The model under review builds one solid part; all positions refer to its coordinate system, in mm. A direction names the side the tool comes from. Coordinates: 2 decimals unless noted, no trailing zeros. Order: outer loops, then holes, each group sorted by start corner. A loop starts at its lowest first (then second) coordinate and runs counter-clockwise, first axis right, second up. Notation, with made-up numbers: (63.25, -10.5) -> (94.25, -10.5) arc R19 ccw to (94.25, 25.5) -> close; hole circle Ø7 at (24.5, 88.5). An arc over 180 degrees is marked (long way). Put each result on its own line as item: value.
Autodesk Inventor part; units mm, degrees
ref_plane "YZ Plane" through (0, 0, 0) normal (1, 0, 0) x (0, 1, 0)
ref_plane "XZ Plane" through (0, 0, 0) normal (0, 1, 0) x (-1, 0, 0)
ref_plane "XY Plane" through (0, 0, 0) normal (0, 0, 1) x (1, 0, 0)
sketch "Sketch1" plane through (0, 0, 0) normal (0, 0, 1) x (1, 0, 0)
  line L0 (-50, 7.5) -> (50, 7.5)
  line L1 (50, 7.5) -> (50, -7.5)
  line L2 (50, -7.5) -> (-50, -7.5)
  line L3 (-50, -7.5) -> (-50, 7.5)
  line L4 (-50, 7.5) -> (50, -7.5) construction
  line L5 (50, 7.5) -> (-50, -7.5) construction
  point P0 (0, 0)
  dimension "d0" = 100
  dimension "d1" = 15
extrude "Extrusion1" add sketch "Sketch1" along normal blind 20
sketch "Sketch2" plane through (-50, -7.5, 0) normal (-1, 0, 0) x (0, 0, 1)
  line L0 (0, 0) -> (0, 15)
  line L1 (0, 0) -> (20, 0)
  line L2 (20, 0) -> (20, 15)
  line L3 (20, 0) -> (20, 6)
  line L4 (11, 15) -> (9, 15)
  line L5 (0, 6) -> (0, 0)
  arc A0 (9, 15) -> (0, 6) centre (9, 6) ccw
  arc A1 (20, 6) -> (11, 15) centre (11, 6) ccw
  point P0 (0, 7.5)
  dimension "d4" = 9
  dimension "d10" = 20
  dimension "d11" = 15
extrude "Extrusion2" cut sketch "Sketch2" against normal through all keep common part
shell "Shell1" thickness 1 removed faces 1 at (-50, 1.5, 10.3333)
extrude "Extrusion3" add sketch "Sketch2" against normal blind 1
sketch "Sketch3" plane through (0, 0, 20) normal (0, 0, 1) x (1, 0, 0)
  line L0 (-50, -7.5) -> (50, -7.5) construction
  line L1 (-50, -7.5) -> (0, -7.5) construction
  line L2 (-50, -7.5) -> (-45, -7.5) construction
  line L3 (-45, -7.5) -> (-45, 7.5) construction
  line L4 (-49, 6.5) -> (49, 6.5) construction
  circle A0 centre (-45, 0) radius 0.25
  line L5 (-45, 0) -> (-15, 0) construction
  circle A1 centre (-15, 0) radius 0.25
  line L6 (-15, 0) -> (15, 0) construction
  circle A2 centre (15, 0) radius 0.25
  line L7 (15, 0) -> (45, 0) construction
  circle A3 centre (45, 0) radius 0.25
  point P0 (0, 0)
  dimension "d12" = 5
  dimension "d13" = 0.5
  dimension "d14" = 30
  dimension "d15" = 0.5
  dimension "d16" = 7.5
  dimension "d17" = 30
  dimension "d18" = 0.5
  dimension "d19" = 30
  dimension "d20" = 0.5
extrude "Extrusion4" cut sketch "Sketch3" against normal through all
properties part number "actuator_tube"
Item 1: Consider section B-B on x = 42. Write out the cut boundary in (y, z).
Answers below:
outline: (-7.5, 0) -> (-1.5, 0) arc R9 ccw to (7.5, 9) -> (7.5, 11) arc R9 ccw to (-1.5, 20) -> (-7.5, 20) -> close; hole (-6.5, 1) -> (-1.5, 1) arc R8 ccw to (6.5, 9) -> (6.5, 11) arc R8 ccw to (-1.5, 19) -> (-6.5, 19) -> close
Item 2: For faces 4 (the flat face through (-1, -4, 19)), 5 (the flat face through (1, -7.5, 10)), list the 3-axis set-ups (+Z, -Z, +X, -X, +Y, -Y) from which the entire face can be reached by the end or side of a thin tool; tool diameter is ignored.
Answers below:
face 4: none
face 5: +Z, -Z, +X, -X, -Y
Item 3: Mouldability with a two-part tool opening along Z and no side actions: class faces 1 (the cylindrical face through (-0.7, 4.934, 2.706)), 2 (the flat face through (50, 0, 10)), 3 (the flat face through (-1, 6.5, 10)) as +Z half, -Z half, draft (parallel to the pull), parting line (faces both ways), or undercut.
Answers below:
face 1: -Z half
face 2: draft
face 3: undercut
Item 4: Consider section C-C on z = 5. Write out the cut boundary in (x, y), and give its area (3 significant figures).
Answers below:
outline: (-50, -7.5) -> (50, -7.5) -> (50, 6.56) -> (-50, 6.56) -> close; hole (-49, -6.5) -> (49, -6.5) -> (49, 5.43) -> (-49, 5.43) -> close
area: 237 mm^2
Item 5: For pin 1 Ø4 at (x, y) = (25, 3.5) entering from -Z; pin 2 Ø6 at (x, z) = (-23, 4.5) entering from +Y; pin 3 Ø6 at (x, y) = (-14.5, 0.5) entering from -Z, all flat-tipped, find the tip position at first contact; note any pin that passes through.
Answers below:
pin 1: z = 0.51
pin 2: y = 7.37
pin 3: z = 0
Item 6: Consider section A-A on y = -3. Write out the cut boundary in (x, z).
Answers below:
outline: (-50, 0) -> (50, 0) -> (50, 20) -> (-50, 20) -> close; hole (-49, 1) -> (49, 1) -> (49, 19) -> (-49, 19) -> close
Item 7: For line 1 (X direction, y = 0, z = 19.2); line 2 (X direction, y = -0.75, z = 7.5); line 3 (Z direction, x = 5, y = -2.75), list the stretches that pass through material, from the lowest coordinate up. Write a range as from..to.
Answers below:
line 1: -50..-45.25, -44.75..-15.25, -14.75..14.75, 15.25..44.75, 45.25..50
line 2: -50..-49, 49..50
line 3: 0..1, 19..20
